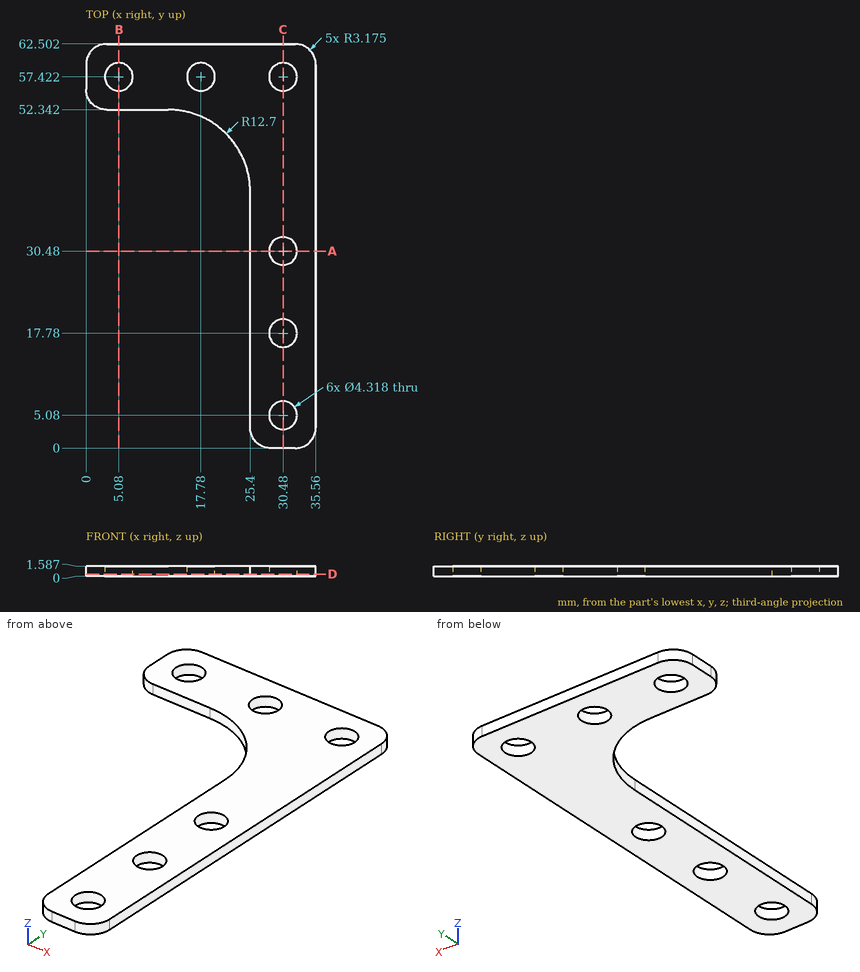
Job drawing, mm, ordinate dimensions from the low corner. One solid piece. Coordinates: 2 decimals unless noted, no trailing zeros. Loops run counter-clockwise (first coordinate to the right, second up) from the corner with the lowest first, then second, coordinate; pieces in that order, holes last. Notation, with made-up numbers: (-14, 31.5) - (10, 31.5) arc R9 cw to (10, 43.5) - close; hole circle Ø4 at (-1, 68.25). An arc over 180 degrees is marked (long way). Answer as a JSON object with one key per item and string values. Group by question number.
(1) Cut at A-A (y = 30.48). Give the cut face in (x, z).
(2) Flat gauge pins, fed straight in: pin 1 (0.5 mm diameter, centred on x = 8, z = 0.5, fed in from -Y); pin 2 (2 mm diameter, centred on x = 28, y = 35, fed in from -Z); pin 3 (0.8 mm diameter, centred on y = 23, z = 0.5, fed in from -X). Where does each tip first touch, or does it go through?
(3) Cut at C-C (x = 30.48). Give the cut face in (y, z).
(4) Cut at B-B (x = 5.08). Give the cut face in (y, z).
(5) Probe line 1 along Y through (x, z) = (30.48, 1.2); line 2 along Y through (x, z) = (5, 0.65) (1 decimal); line 3 along X through (y, z) = (22, 1.45). List the from-to ranges inside material, lowest first.
(6) Cut at D-D (z = 0.35). State how many separate pieces and enclosed holes the cut face has, then the cut area to 3 significant figures.
Geometry says:
{
 "1": {"outline": "(25.4, 0) - (28.32, 0) - (28.32, 1.59) - (25.4, 1.59) - close; (32.64, 0) - (35.56, 0) - (35.56, 1.59) - (32.64, 1.59) - close"},
 "2": {"pin 1": "stops at y = 52.34", "pin 2": "stops at z = 0", "pin 3": "stops at x = 25.4"},
 "3": {"outline": "(0, 0) - (2.92, 0) - (2.92, 1.59) - (0, 1.59) - close; (7.24, 0) - (15.62, 0) - (15.62, 1.59) - (7.24, 1.59) - close; (19.94, 0) - (28.32, 0) - (28.32, 1.59) - (19.94, 1.59) - close; (32.64, 0) - (55.26, 0) - (55.26, 1.59) - (32.64, 1.59) - close; (59.58, 0) - (62.5, 0) - (62.5, 1.59) - (59.58, 1.59) - close"},
 "4": {"outline": "(52.34, 0) - (55.26, 0) - (55.26, 1.59) - (52.34, 1.59) - close; (59.58, 0) - (62.5, 0) - (62.5, 1.59) - (59.58, 1.59) - close"},
 "5": {"line 1": "y = 0 to 2.92, 7.24 to 15.62, 19.94 to 28.32, 32.64 to 55.26, 59.58 to 62.5", "line 2": "y = 52.3 to 55.3, 59.6 to 62.5", "line 3": "x = 25.4 to 35.56"},
 "6": {"separate pieces": "1", "enclosed holes": "6", "area": "829 mm^2"}
}
